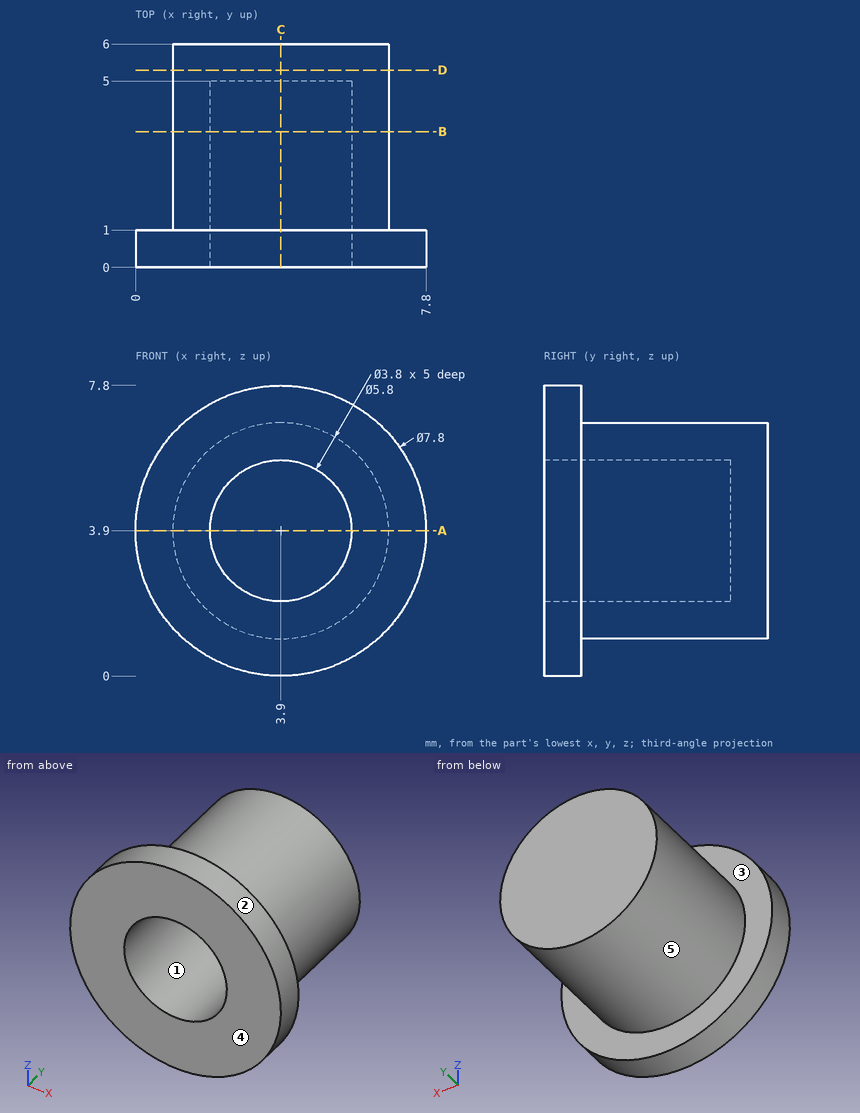
Source: three-view drawing plus pictorial views. Frame: mm from the lowest corner of the part. A direction names the side the tool comes from. Round coordinates to 2 decimals unless told otherwise and drop trailing zeros. Loops run counter-clockwise (first coordinate to the right, second up) from the corner with the lowest first, then second, coordinate; pieces in that order, holes last. Notation, with made-up numbers: (54, -10) - (65, -10) arc R12 ccw to (65, -6) - close; hole circle Ø5 at (-17.75, 75). An arc over 180 degrees is marked (long way). Write item = value, one per line. Start each with the question number.
Item 1: Section query A-A on z = 3.9. Output: boundary loops of the cut face in (x, y).
Item 2: Section query B-B on y = 3.65. Output: boundary loops of the cut face in (x, z), plus the area to 3 significant figures.
Item 3: Section query C-C on x = 3.9. Output: boundary loops of the cut face in (y, z).
Item 4: Material intervals for line 1 (X direction, y = 1.3, z = 3.9); line 2 (Y direction, x = 0.75, z = 4.25); line 3 (X direction, y = 0.95, z = 4), sorted ascending.
Item 5: Mould query, pull axis Z, two halves, no side actions, for the marked faces 1, 2 and 3. Classes: released by +Z, released by -Z, zero draft, split by the parting line, or undercut.
Item 6: Section query D-D on y = 5.3. Output: boundary loops of the cut face in (x, z), plus the area to 3 significant figures.
Item 7: First-contact query: pin 1 Ø1.5 at (y, z) = (5, 3) entering from -X; pin 2 Ø2.5 at (x, z) = (3.9, 3.9) entering from -Y; pin 3 Ø1 at (x, y) = (4.5, 3) entering from -Z. Flat tips, straight axial feed; report the tip coordinate or a pass-through.
Item 8: Reachability of the marked faces 4 and 5 from +Z, -Z, +X, -X, +Y, -Y: full face, straight path, thin tool, end or side. Return the list, or none.
Results list:
q1.outline = (0, 0) - (2, 0) - (2, 5) - (5.8, 5) - (5.8, 0) - (7.8, 0) - (7.8, 1) - (6.8, 1) - (6.8, 6) - (1, 6) - (1, 1) - (0, 1) - close
q2.outline = circle Ø5.8 at (3.9, 3.9); hole circle Ø3.8 at (3.9, 3.9)
q2.area = 15.1 mm²
q3.outline = (0, 0) - (1, 0) - (1, 1) - (6, 1) - (6, 6.8) - (1, 6.8) - (1, 7.8) - (0, 7.8) - (0, 5.8) - (5, 5.8) - (5, 2) - (0, 2) - close
q4.line_1 = 1 to 2, 5.8 to 6.8
q4.line_2 = 0 to 1
q4.line_3 = 0 to 2, 5.8 to 7.8
q5.face_1 = undercut
q5.face_2 = split by the parting line
q5.face_3 = zero draft
q6.outline = circle Ø5.8 at (3.9, 3.9)
q6.area = 26.4 mm²
q7.pin_1 = 1
q7.pin_2 = 5
q7.pin_3 = 1
q8.face_4 = +Z, -Z, +X, -X, -Y
q8.face_5 = +Y
